```python
from build123d import *

# Parameters (mm, degrees)
EXTRUDE_1_DEPTH     = 1
SKETCH_2_W          = 89.659893576
SKETCH_2_H          = 2
CUT_EXTRUDE_1_DEPTH = 10


with BuildPart() as part:
    # 草图1 → 凸台-拉伸1 (new, symmetric)
    with BuildSketch(Plane(origin=(0, 0, 0), x_dir=(1, 0, 0), z_dir=(0, 1, 0))):
        with BuildLine():
            Line((55, 0), (-55, 0))
            Line((-55, 0), (-55, 90))
            Line((-55, 90), (-40, 147.411542732))
            Line((-40, 147.411542732), (-40, 159.411542732))
            Line((-40, 159.411542732), (-49.788880489, 162.334425912))
            ThreePointArc((-49.788880489, 162.334425912), (-55.499718249, 170.067141222), (-49.659893575, 177.70291242))
            Line((-49.659893575, 177.70291242), (-40, 180.411542732))
            Line((-40, 180.411542732), (-40, 194.411542732))
            Line((-40, 194.411542732), (-31, 210))
            Line((-31, 210), (31, 210))
            Line((31, 210), (40, 194.411542732))
            Line((40, 194.411542732), (40, 180.411542732))
            Line((40, 180.411542732), (49.659893575, 177.70291242))
            ThreePointArc((49.659893575, 177.70291242), (55.499718249, 170.067141222), (49.788880489, 162.334425912))
            Line((49.788880489, 162.334425912), (40, 159.411542732))
            Line((40, 159.411542732), (40, 147.411542732))
            Line((40, 147.411542732), (55, 90))
            Line((55, 90), (55, 0))
        make_face()
    extrude(amount=EXTRUDE_1_DEPTH, both=True)

    # 草图2 → 切除-拉伸1 (cut)
    with BuildSketch(Plane(origin=(0, 0, -210), x_dir=(-1, 0, 0), z_dir=(0, 0, -1))):
        Rectangle(SKETCH_2_W, SKETCH_2_H)
    extrude(amount=-CUT_EXTRUDE_1_DEPTH, mode=Mode.SUBTRACT)


solid = part.part
```
Read the model definition and answer for the solid it produces. Units are mm, in the model's axes. A direction names the side the tool comes from. Coordinates: 2 decimals unless noted, no trailing zeros. Write each loop counter-clockwise with the first axis right and the second up, starting at its lowest first coordinate (ties: lowest second). Pieces come first, ordered by that corner, then holes. Notation, with made-up numbers: (-31.75, -13.75) - (18.25, -13.75) arc R13 ccw to (18.25, 5.25) - close; hole circle Ø8 at (40.5, 72). An arc over 180 degrees is marked (long way). Answer as a JSON object with one key per item and string values. Group by question number.
1. This flat-tipped pin is pushed along its axis until it touches: P1, Ø1, axis at y = 0, z = -186.5, coming from the +X side. Where does it stop, or does it pass through?
2. Which of the six approach directions +Z, -Z, +X, -X, +Y, -Y give full straight-line access (tool end or side, diameter ignored) to faces 1 (the flat face through (-47.605, 0.014, -118.304)), 2 (the cylindrical face through (55.497, 0.014, -170.211))?
3. A cutting plane is placed at A-A (y = 0.5). Determine the outline of the cut face in (x, z).
4. The mould has two halves that part along Z. Classify faces 3 (the flat face through (1, 1, -101)), 4 (the flat face through (47.395, 0.014, -119.108)): +Z half, -Z half, draft (parallel to the pull), parting line (faces both ways), or undercut.
5. A cutting plane is placed at B-B (z = -93.5). Determine the outline of the cut face in (x, y), plus the area to 3 significant figures.
6. Consider L1, parallel to X at y = -0.7, z = -11; L2, parallel to X at y = 0.25, z = -164. Determine where each line is inside the solid, lowest interval first. Write a range as [from, to].
7. A cutting plane is placed at C-C (z = -166). Determine the outline of the cut face in (x, y), plus the area to 3 significant figures.
Worked out:
{
 "1": {"P1": "stops at x = 40"},
 "2": {"face 1": "-X, +Y, -Y", "face 2": "+X, +Y, -Y"},
 "3": {"outline": "(-55, -90) - (-40, -147.41) - (-40, -159.41) - (-49.79, -162.33) arc R8 ccw to (-49.66, -177.7) - (-40, -180.41) - (-40, -194.41) - (-36.77, -200) - (36.77, -200) - (40, -194.41) - (40, -180.41) - (49.66, -177.7) arc R8 ccw to (49.79, -162.33) - (40, -159.41) - (40, -147.41) - (55, -90) - (55, 0) - (-55, 0) - close"},
 "4": {"face 3": "draft", "face 4": "undercut"},
 "5": {"outline": "(-54.09, -1) - (54.09, -1) - (54.09, 1) - (-54.09, 1) - close", "area": "216 mm²"},
 "6": {"L1": "x = [-55, 55]", "L2": "x = [-52.79, 52.79]"},
 "7": {"outline": "(-54.43, -1) - (54.43, -1) - (54.43, 1) - (-54.43, 1) - close", "area": "218 mm²"}
}
